Read the model definition and answer for the solid it produces. Units are mm, in the model's axes. A direction names the side the tool comes from. Give positions to 0.01 mm unless a question says otherwise; leave off trailing zeros. Order: outer loops, then holes, each group sorted by start corner. A loop starts at its lowest first (then second) coordinate and runs counter-clockwise, first axis right, second up. Notation, with made-up numbers: M 56.5,2.25 L 71.5,2.25 A19 cw 71.5,19.25 Z; hole C -17.5,-12 d11. An arc over 180 degrees is marked long. One line per item, written item: value.
from build123d import *

# Parameters (mm, degrees)
MAIN_DEPTH                         = 10
ESQUISSE4_W                        = 2.9
ESQUISSE4_H                        = 40
MAKERBEAMFIXVERTICAL_DEPTH         = 1
MAKERBEAMVERTICALHOLE_DEPTH        = 58.445626465
MAKERBEAMVERTICALHOLE_DEPTH_BACK   = 58.445626465
ESQUISSE2_R                        = 1.5
ESQUISSE5_W                        = 40
ESQUISSE5_H                        = 2.9
MAKERBEAMFIXHORIZONTAL_DEPTH       = 1
MAKERBEAMHORIZONTALHOLE_DEPTH      = 58.445626465
MAKERBEAMHORIZONTALHOLE_DEPTH_BACK = 58.445626465
ESQUISSE3_R                        = 1.5
BOSS_EXTRUDE1_DEPTH                = 10
FILLET1_R                          = 1


with BuildPart() as part:
    # Esquisse1 → Main (new body)
    with BuildSketch(Plane.XY):
        with BuildLine():
            Line((0, 0), (40, 0))
            Line((40, 0), (40, 5))
            Line((40, 5), (9, 5))
            ThreePointArc((9, 5), (6.171572875, 6.171572875), (5, 9))
            Line((5, 9), (5, 40))
            Line((5, 40), (0, 40))
            Line((0, 40), (0, 0))
        make_face()
    extrude(amount=MAIN_DEPTH)

    # Esquisse4 → MakerBeamFixVertical (add)
    with BuildSketch(Plane.ZY):
        with Locations((5, 20)):
            Rectangle(ESQUISSE4_W, ESQUISSE4_H)
    extrude(amount=MAKERBEAMFIXVERTICAL_DEPTH)

    # Esquisse2 → MakerBeamVerticalHole (cut, two sides: drawn at the far end of the back side and taken through both)
    with BuildSketch(Plane.ZY.offset(-MAKERBEAMVERTICALHOLE_DEPTH_BACK)):
        with Locations(Location((5, 35, 0), (0, 0, 270))):
            Circle(ESQUISSE2_R)
    extrude(amount=MAKERBEAMVERTICALHOLE_DEPTH + MAKERBEAMVERTICALHOLE_DEPTH_BACK, mode=Mode.SUBTRACT)

    # Esquisse5 → MakerBeamFixHorizontal (add)
    with BuildSketch(Plane(origin=(0, 0, 0), x_dir=(-1, 0, 0), z_dir=(0, -1, 0))):
        with Locations((-20, -5)):
            Rectangle(ESQUISSE5_W, ESQUISSE5_H)
    extrude(amount=MAKERBEAMFIXHORIZONTAL_DEPTH)

    # Esquisse3 → MakerBeamHorizontalHole (cut, two sides: drawn at the far end of the back side and taken through both)
    with BuildSketch(Plane.XZ.offset(-MAKERBEAMHORIZONTALHOLE_DEPTH_BACK)):
        with Locations(Location((35, 5, 0), (0, 0, 255.164888418))):
            Circle(ESQUISSE3_R)
    extrude(amount=MAKERBEAMHORIZONTALHOLE_DEPTH + MAKERBEAMHORIZONTALHOLE_DEPTH_BACK, mode=Mode.SUBTRACT)

    # Sketch2 → Boss-Extrude1 (add)
    with BuildSketch(Plane.XY.offset(10)):
        Polygon((5, 30), (30, 5), (22, 5), (5, 22), align=None)
    extrude(amount=-BOSS_EXTRUDE1_DEPTH)

    # Fillet1
    fillet1_edges = [part.edges().sort_by_distance(p)[0] for p in [
        (5, 22, 5),
        (5, 30, 5),
        (30, 5, 5),
        (22, 5, 5),
    ]]
    fillet(fillet1_edges, radius=FILLET1_R)


solid = part.part
1) Determine the mould class of faces 5 (the face through (20, 0, 8)), 6 (the face through (5, 36.2, 3.8)), 7 (the face through (6.203, 6.141, 4.93)), 8 (the face through (5, 14, 5)) for opening direction Y: +Y half, -Y half, draft (parallel to the pull), parting line (faces both ways), or undercut.
Reported:
face 5: -Y half
face 6: draft
face 7: undercut
face 8: undercut
2) Which of the six approach directions +Z, -Z, +X, -X, +Y, -Y give full straight-line access (tool end or side, diameter ignored) to faces 1 (the face through (-0.5, 37.7, 3.55)), 2 (the face through (0, -0.5, 5)), 3 (the face through (-0.5, 37.7, 6.45)), 4 (the face through (37.7, -0.5, 3.55))?
Reported:
face 1: -Z, -X, +Y, -Y
face 2: +Z, -Z, -X, -Y
face 3: +Z, -X, +Y, -Y
face 4: -Z, +X, -X, -Y
3) Find section A-A, the plane z = 5. Write down the section's boundary in (x, y).
Reported:
outline: M -1,0 L 0,0 L 0,-1 L 33.5,-1 L 33.5,5 L 30.41,5 A1 cw 29.71,5.29 L 5.29,29.71 A1 cw 5,30.41 L 5,33.5 L -1,33.5 Z; M -1,36.5 L 5,36.5 L 5,40 L -1,40 Z; M 36.5,-1 L 40,-1 L 40,5 L 36.5,5 Z; hole M 5,9 A4 ccw 9,5 L 19.59,5 A1 ccw 20.29,6.71 L 6.71,20.29 A1 ccw 5,19.59 Z
4) Each of these flat-tipped pins is pushed along its axis until it touches: pin 1 Ø1.1 at (x, z) = (13, 8) entering from -Y; pin 2 Ø4 at (y, z) = (10, 1.5) entering from +X; pin 3 Ø2.5 at (x, z) = (35, 5) entering from -Y; pin 4 Ø5 at (x, z) = (13, 6.5) entering from +Y. Where does it stop, or does it pass through?
Reported:
pin 1: stops at y = 0
pin 2: stops at x = 27
pin 3: passes through
pin 4: stops at y = 24.5
5) Find section C-C, the plane y = 17.5. Write down the section's boundary in (x, z), plus the area to 3 significant figures.
Reported:
outline: M -1,3.55 L 0,3.55 L 0,0 L 5,0 L 5,10 L 0,10 L 0,6.45 L -1,6.45 Z; M 9.5,0 L 17.5,0 L 17.5,10 L 9.5,10 Z
area: 133 mm^2
6) Find section B-B, the plane x = 13. Write down the section's boundary in (y, z), plus the area to 3 significant figures.
Reported:
outline: M -1,3.55 L 0,3.55 L 0,0 L 5,0 L 5,10 L 0,10 L 0,6.45 L -1,6.45 Z; M 14,0 L 22,0 L 22,10 L 14,10 Z
area: 133 mm^2
7) Find section D-D, the plane x = 4. Write down the section's boundary in (y, z), plus the area to 3 significant figures.
Reported:
outline: M -1,3.55 L 0,3.55 L 0,0 L 40,0 L 40,10 L 0,10 L 0,6.45 L -1,6.45 Z; hole C 35,5 d3
area: 396 mm^2
8) Consider probe 1 along Z at (x, y) = (35, 2.9); probe 2 along X at (y, z) = (2.7, 5). Determine where each line is inside the solid, lowest interval first.
Reported:
probe 1: z = 0 to 3.5, 6.5 to 10
probe 2: x = -1 to 33.5, 36.5 to 40
